```python
from build123d import *

# Parameters (mm, degrees)
BOSS_EXTRUDE1_DEPTH = 3
SKETCH2_R           = 4.1656
CUT_EXTRUDE1_DEPTH  = 158.283042746
SKETCH3_W           = 10.000000066
SKETCH3_H           = 3
CUT_EXTRUDE2_DEPTH  = 158.283042746


with BuildPart() as part:
    # Sketch1 → Boss-Extrude1 (new body)
    with BuildSketch(Plane(origin=(0, 0, 0), x_dir=(-1, 0, 0), z_dir=(0, 0, 1))):
        with BuildLine():
            Line((16.6878, -36.83), (54.810334268, -36.83))
            ThreePointArc((54.810334268, -36.83), (56.606385492, -36.086051224), (57.350334268, -34.29))
            Line((57.350334268, -34.29), (57.350334268, 77.47))
            Line((57.350334268, 77.47), (82.750334268, 95.25))
            Line((82.750334268, 95.25), (82.750334268, 133.721119177))
            ThreePointArc((82.750334268, 133.721119177), (43.408002592, 116.840177161), (3.980183448, 133.520475199))
            Line((3.980183448, 133.520475199), (3.980183448, 119.349325812))
            Line((3.980183448, 119.349325812), (29.380183448, 101.564054342))
            Line((29.380183448, 101.564054342), (29.380183448, 90.17))
            Line((29.380183448, 90.17), (29.380183448, 13.97))
            Line((29.380183448, 13.97), (16.680183448, 13.97))
            Line((16.680183448, 13.97), (16.680183448, 1.27))
            Line((16.680183448, 1.27), (19.250334268, -1.27))
            Line((19.250334268, -1.27), (19.250334268, -34.29))
            Line((19.250334268, -34.29), (16.6878, -36.83))
        make_face()
    extrude(amount=BOSS_EXTRUDE1_DEPTH)

    # Sketch2 → Cut-Extrude1 (cut, through all)
    with BuildSketch(Plane.XY.offset(3)):
        with Locations((-38.300334268, 17.78)):
            Circle(SKETCH2_R)
    extrude(amount=-CUT_EXTRUDE1_DEPTH, mode=Mode.SUBTRACT)

    # Sketch3 → Cut-Extrude2 (cut, through all)
    with BuildSketch(Plane.XY.offset(3)):
        with Locations((-49.602137137, -106.461390659)):
            Rectangle(SKETCH3_W, SKETCH3_H)
    extrude(amount=-CUT_EXTRUDE2_DEPTH, mode=Mode.SUBTRACT)


solid = part.part
```
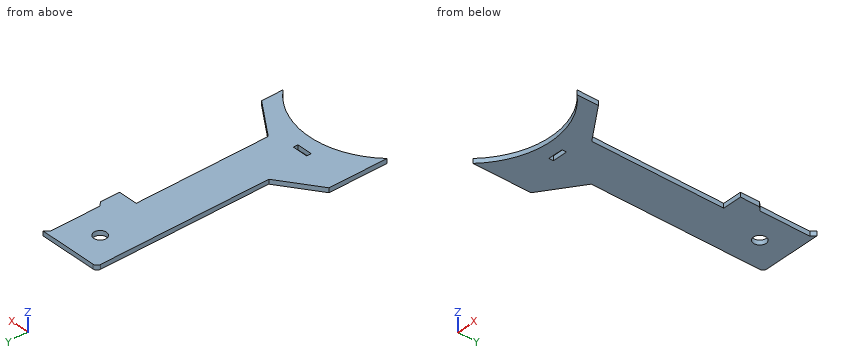
Check sheet for the modelled part. Datum: model origin and axes. Units: mm. Give positions to 0.01 mm unless a question says otherwise; leave off trailing zeros. Order: outer loops, then holes, each group sorted by start corner. A loop starts at its lowest first (then second) coordinate and runs counter-clockwise, first axis right, second up. Notation, with made-up numbers: M -20.5,47 L 13.5,47 A28 cw 13.5,75 Z; hole C 34,-39 d9. An arc over 180 degrees is marked long. Answer in a Markdown table with one row per item.
1) Cross-section at B-B, the plane x = -38.5. Enter the section's corners in (y, z), plus the area to 3 significant figures.
Filled sheet:
| item | result |
|---|---|
| outline | M -117.05,0 L 13.62,0 L 13.62,3 L -117.05,3 Z; M 21.94,0 L 36.83,0 L 36.83,3 L 21.94,3 Z |
| area | 437 mm2 |
2) Cross-section at D-D, the plane y = -86. Enter the section's corners in (x, z).
Filled sheet:
| item | result |
|---|---|
| outline | M -69.54,0 L -29.38,0 L -29.38,3 L -69.54,3 Z |
3) Cross-section at A-A, the plane y = 17.78. Enter the section's corners in (x, z).
Filled sheet:
| item | result |
|---|---|
| outline | M -57.35,0 L -42.47,0 L -42.47,3 L -57.35,3 Z; M -34.13,0 L -19.25,0 L -19.25,3 L -34.13,3 Z |
4) Cross-section at C-C, the plane z = 1.1. Enter the section's corners in (x, y).
Filled sheet:
| item | result |
|---|---|
| outline | M -82.75,-133.72 A54.61 cw -3.98,-133.52 L -3.98,-119.35 L -29.38,-101.56 L -29.38,-13.97 L -16.68,-13.97 L -16.68,-1.27 L -19.25,1.27 L -19.25,34.29 L -16.69,36.83 L -54.81,36.83 A2.54 ccw -57.35,34.29 L -57.35,-77.47 L -82.75,-95.25 Z; hole M -54.6,-107.96 L -44.6,-107.96 L -44.6,-104.96 L -54.6,-104.96 Z; hole C -38.3,17.78 d8.33 |
5) Thickness scan on L1, parallel to X at y = -98, z = 0.85; L2, parallel to Y at x = -46, z = 2.05; L3, parallel to Y at x = -27, z = 2.4. Record the ranges inside material, lowest first. Write a range as [from, to].
Filled sheet:
| item | result |
|---|---|
| L1 | x = [-82.75, -29.38] |
| L2 | y = [-116.91, -107.96], [-104.96, 36.83] |
| L3 | y = [-119.32, -103.23], [-13.97, 36.83] |
6) Gauge pin test, flat ends, axial feed: P1, Ø1.5, axis at y = -106.5, z = 1, coming from the +X side; P2, Ø0.9, axis at y = -38, z = 1, coming from the +X side; P3, Ø1.5, axis at y = -9.5, z = 1.5, coming from the +X side. Record the tip position at first contact, or that the pin passes through.
Filled sheet:
| item | result |
|---|---|
| P1 | stops at x = -21.26 |
| P2 | stops at x = -29.38 |
| P3 | stops at x = -16.68 |
